from build123d import *

# Parameters (mm, degrees)
F1_DEPTH      = 28.575
F2_W          = 69.85
F2_H          = 1.5875
F3_DEPTH      = 69.85
F6_DEPTH      = 1.5875
F6_DEPTH_BACK = 1.5875
F7_R          = 1.58749


# Not quite as in the source:
# - a fillet or chamfer is up to 0.001 mm smaller than in the source, because OpenCascade refuses the exact size


with BuildPart() as f1:
    # F0 (on Top) → F1 (new body)
    with BuildSketch(Plane.XY):
        Polygon((53.975, -34.925), (53.975, 0), (53.975, 34.925), (-53.975, 34.925), (-53.975, -34.925), align=None)
    extrude(amount=F1_DEPTH)

    # F2 (on face) → F3 (cut, through all)
    with BuildSketch(Plane.XZ.offset(34.925)):
        with Locations((-9.525, 16.66875)):
            Rectangle(F2_W, F2_H)
    extrude(amount=-F3_DEPTH, mode=Mode.SUBTRACT)

    # F5 (on offset) → F6 (join, two sides)
    with BuildSketch(Plane.XZ.offset(-1.5875)) as f6_sk:
        Polygon((53.975, 19.05), (53.975, 15.875), (71.4375, 15.875), (71.4375, 3.175), (90.4875, 3.175), (90.4875, 6.35), (74.6125, 6.35), (74.6125, 19.05), align=None)
    extrude(amount=F6_DEPTH)
    extrude(f6_sk.sketch, amount=-F6_DEPTH_BACK)

    # F7 (radius 1.5875 in the source; OpenCascade refuses exactly that, so slightly less here)
    f7_edges = [f1.edges().sort_by_distance(p)[0] for p in [
        (64.29375, 0, 19.05),
        (74.6125, 3.175, 12.7),
        (74.6125, 0, 12.7),
        (74.6125, 1.5875, 19.05),
        (74.6125, 1.5875, 6.35),
        (71.4375, 0, 9.525),
        (62.70625, 0, 15.875),
        (64.29375, 3.175, 19.05),
        (82.55, 3.175, 6.35),
        (82.55, 0, 6.35),
        (80.9625, 0, 3.175),
        (90.4875, 1.5875, 3.175),
        (90.4875, 0, 4.7625),
        (90.4875, 1.5875, 6.35),
        (90.4875, 3.175, 4.7625),
        (62.70625, 3.175, 15.875),
        (71.4375, 1.5875, 3.175),
        (80.9625, 3.175, 3.175),
        (71.4375, 3.175, 9.525),
        (71.4375, 1.5875, 15.875),
    ]]
    fillet(f7_edges, radius=F7_R)


solid = f1.part
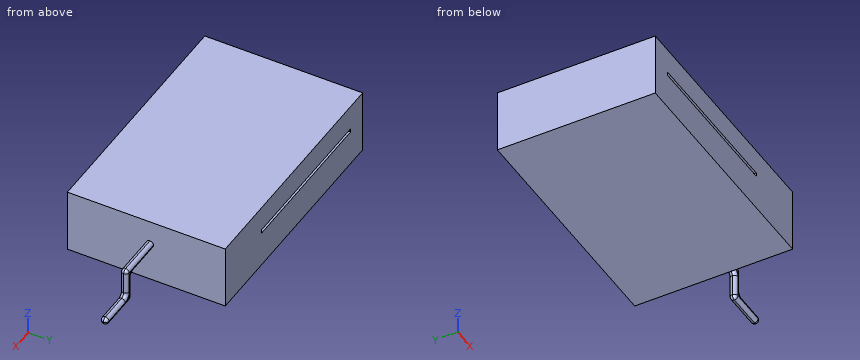
Design review of the part built by this model. Coordinates are the model's own, in mm. Coordinates: 2 decimals unless noted, no trailing zeros. Order: outer loops, then holes, each group sorted by start corner. A loop starts at its lowest first (then second) coordinate and runs counter-clockwise, first axis right, second up.
Item 1: For line 1 (Z direction, x = -41, y = -27.5) (1 decimal); line 2 (X direction, y = -28.5, z = 16) (3 decimals); line 3 (X direction, y = -25.5, z = 21.75) (3 decimals), list the stretches that pass through material, from the lowest coordinate up.
Item 2: Take a section at C-C, the plane x = 16.5. Write out the cut boundary in (y, z) (1 decimal), then the cut area to 3 significant figures.
Item 3: For pin 1 Ø1.7 at (y, z) = (17, 17) entering from +X (3 decimals); pin 2 Ø8 at (x, y) = (35.5, -12.5) entering from -Z; pin 3 Ø14 at (x, z) = (73.5, 10.5) entering from -Y, all flat-tipped, find the tip position at first contact; note any pin that passes through.
The answers:
1. line 1: z = 0 to 15.9, 17.5 to 28.6
1. line 2: x = -53.975 to -44.45, 25.4 to 53.975
1. line 3: x = -53.975 to 53.975
2. outline: (-34.9, 0) - (34.9, 0) - (34.9, 15.9) - (-34.9, 15.9) - close; (-34.9, 17.5) - (34.9, 17.5) - (34.9, 28.6) - (-34.9, 28.6) - close
2. area: 1,890 mm2
3. pin 1: stops at x = 53.975
3. pin 2: stops at z = 0
3. pin 3: stops at y = 0
